Can you work these out from the drawing? Everything is in mm from the part's minimum corner. Give positions to 0.01 mm unless a question says otherwise; leave off trailing zeros. Write each loop counter-clockwise with the first axis right and the second up, starting at its lowest first coordinate (ties: lowest second). Pieces come first, ordered by that corner, then holes. Notation, with made-up numbers: (59.25, 58) -> (115.25, 58) arc R23 cw to (115.25, 92) -> close; hole circle Ø4 at (28, 19.25). An arc over 180 degrees is marked (long way). Answer as CSV lines item,"result". Start each with the question number.
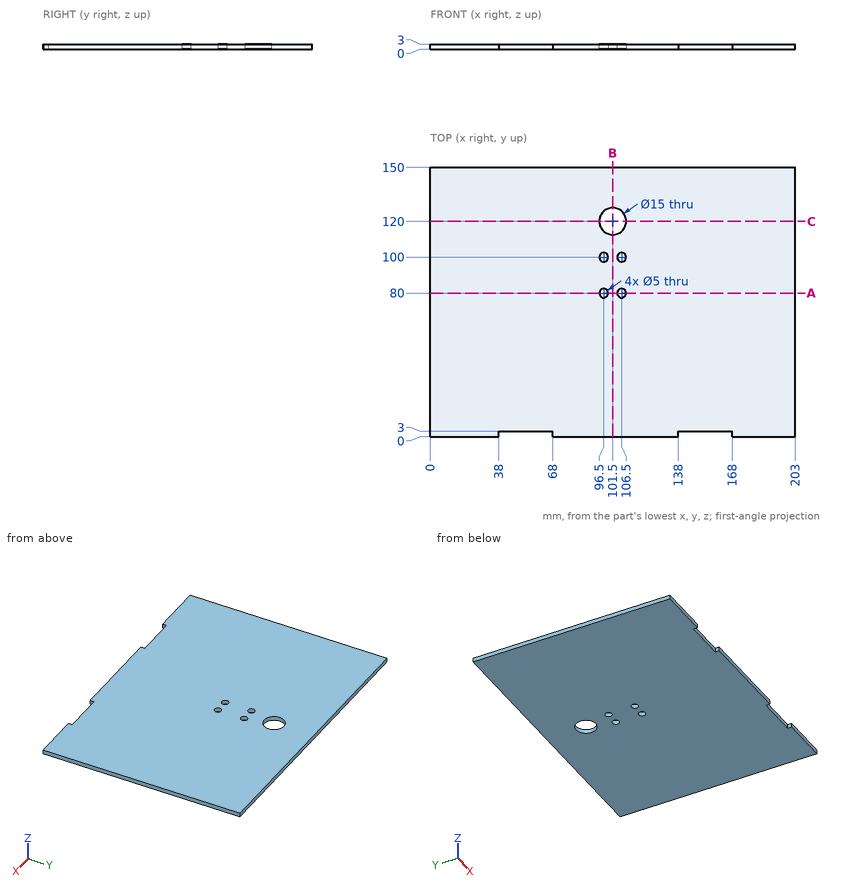
Item 1: If we section it at B-B (x = 101.5): Please give me the cut outline in (y, z), and give its area (3 significant figures).
Item 2: If I drill on line 1 (Y direction, x = 106.5, z = 2.3); line 2 (Y direction, x = 101.5, z = 1.4); line 3 (Y direction, x = 144, z = 0.8), over which ranges is the centre line in solid material (lowest first)? Write a range as [from, to].
Item 3: If we section it at C-C (y = 120): Please give me the cut outline in (x, z).
Item 4: I'm going to push a flat-ended pin straight in: pin 1 (4.5 mm diameter, centred on x = 96.5, y = 80, fed in from -Z). Where does the tip first touch, or does it pass through?
Item 5: If we section it at A-A (y = 80): Please give me the cut outline in (x, z), and give its area (3 significant figures).
Final values:
1,outline,"(0, 0) -> (112.5, 0) -> (112.5, 3) -> (0, 3) -> close; (127.5, 0) -> (150, 0) -> (150, 3) -> (127.5, 3) -> close"
1,area,"405 mm2"
2,line 1,"[0, 77.5], [82.5, 97.5], [102.5, 114.41], [125.59, 150]"
2,line 2,"[0, 112.5], [127.5, 150]"
2,line 3,"[3, 150]"
3,outline,"(0, 0) -> (94, 0) -> (94, 3) -> (0, 3) -> close; (109, 0) -> (203, 0) -> (203, 3) -> (109, 3) -> close"
4,pin 1,"through"
5,outline,"(0, 0) -> (94, 0) -> (94, 3) -> (0, 3) -> close; (99, 0) -> (104, 0) -> (104, 3) -> (99, 3) -> close; (109, 0) -> (203, 0) -> (203, 3) -> (109, 3) -> close"
5,area,"579 mm2"
